CAD build for the part. Positions are in the model's coordinates, mm. A direction names the side the tool comes from. Round coordinates to 2 decimals unless told otherwise and drop trailing zeros. Loops run counter-clockwise (first coordinate to the right, second up) from the corner with the lowest first, then second, coordinate; pieces in that order, holes last. Notation, with made-up numbers: M -2,67 L 42,67 A30 cw 42,100 Z; hole C 12,83 d6. An arc over 180 degrees is marked long. Use one line per item in the form item = value.
from build123d import *

# Parameters (mm, degrees)
CROQUIS1_R              = 14
SALIENTE_EXTRUIR1_DEPTH = 3.5
CROQUIS2_R              = 17.2
SALIENTE_EXTRUIR2_DEPTH = 3.2
CROQUIS3_R              = 17.2
SALIENTE_EXTRUIR3_DEPTH = 3.2
CROQUIS4_R              = 1.5
CORTAR_EXTRUIR1_DEPTH   = 10.9
REDONDEO1_R             = 2
REDONDEO2_R             = 0.5


with BuildPart() as part:
    # Croquis1 → Saliente-Extruir1 (new body)
    with BuildSketch(Plane(origin=(0, 0, 0), x_dir=(1, 0, 0), z_dir=(0, 1, 0))):
        Circle(CROQUIS1_R)
    extrude(amount=SALIENTE_EXTRUIR1_DEPTH)

    # Croquis2 → Saliente-Extruir2 (add)
    with BuildSketch(Plane(origin=(0, 3.5, 0), x_dir=(1, 0, 0), z_dir=(0, 1, 0))):
        Circle(CROQUIS2_R)
    extrude(amount=SALIENTE_EXTRUIR2_DEPTH)

    # Croquis3 → Saliente-Extruir3 (add)
    with BuildSketch(Plane.XZ):
        Circle(CROQUIS3_R)
    extrude(amount=SALIENTE_EXTRUIR3_DEPTH)

    # Croquis4 → Cortar-Extruir1 (cut, through all)
    with BuildSketch(Plane.XZ.offset(3.2)):
        Circle(CROQUIS4_R)
    extrude(amount=-CORTAR_EXTRUIR1_DEPTH, mode=Mode.SUBTRACT)

    # Redondeo1
    redondeo1_edges = [part.edges().sort_by_distance(p)[0] for p in [
        (-17.2, 0, 0),
        (-17.2, 3.5, 0),
    ]]
    fillet(redondeo1_edges, radius=REDONDEO1_R)

    # Redondeo2
    redondeo2_edges = [part.edges().sort_by_distance(p)[0] for p in [
        (-14, 0, 0),
        (-14, 3.5, 0),
    ]]
    fillet(redondeo2_edges, radius=REDONDEO2_R)


solid = part.part
1. Probe line 1 along Y through (x, z) = (-7.5, -12.5); line 2 along Z through (x, y) = (0.5, 2.25); line 3 along Z through (x, y) = (0, -1). List the from-to ranges inside material, lowest first. Write a range as from..to.
Completed:
line_1 = -3.2..0, 3.5..6.7
line_2 = -13.99..-1.41, 1.41..13.99
line_3 = -16.93..-1.5, 1.5..16.93
2. Pull direction Z, two halves, no side cores. Call faces 1 (the face through (0, 0, -15)), 2 (the face through (-17.183, -2.592, 0.756)), 3 (the face through (-1.5, 1.68, 0.07)): +Z half, -Z half, draft (parallel to the pull), parting line (faces both ways), or undercut.
Completed:
face_1 = draft
face_2 = parting line
face_3 = undercut
3. Cut at B-B on z = 0. Write the cut outline in (x, y).
Completed:
outline = M -17.2,-3.2 L -1.5,-3.2 L -1.5,6.7 L -17.2,6.7 L -17.2,5.5 A2 ccw -15.2,3.5 L -14.5,3.5 A0.5 cw -14,3 L -14,0.5 A0.5 cw -14.5,0 L -15.2,0 A2 ccw -17.2,-2 Z; M 1.5,-3.2 L 17.2,-3.2 L 17.2,-2 A2 ccw 15.2,0 L 14.5,0 A0.5 cw 14,0.5 L 14,3 A0.5 cw 14.5,3.5 L 15.2,3.5 A2 ccw 17.2,5.5 L 17.2,6.7 L 1.5,6.7 Z
4. Cut at C-C on y = 6. Write the cut outline in (x, z).
Completed:
outline = C 0,0 d34.4; hole C 0,0 d3
5. Drop flat-ended pins along their axis: P1, Ø5, axis at y = -2, z = 10.5, coming from the +X side; P2, Ø5, axis at y = -1, z = 4.5, coming from the +X side; P3, Ø1, axis at y = 5.5, z = -12, coming from the -X side. Give the stop position or say it passes through.
Completed:
P1 = 15.23
P2 = 17.06
P3 = -12.79
6. Cut at A-A on x = 0. Write the cut outline in (y, z), and give its area (3 significant figures).
Completed:
outline = M -3.2,-17.2 L -2,-17.2 A2 ccw 0,-15.2 L 0,-14.5 A0.5 cw 0.5,-14 L 3,-14 A0.5 cw 3.5,-14.5 L 3.5,-15.2 A2 ccw 5.5,-17.2 L 6.7,-17.2 L 6.7,-1.5 L -3.2,-1.5 Z; M -3.2,1.5 L 6.7,1.5 L 6.7,17.2 L 5.5,17.2 A2 ccw 3.5,15.2 L 3.5,14.5 A0.5 cw 3,14 L 0.5,14 A0.5 cw 0,14.5 L 0,15.2 A2 ccw -2,17.2 L -3.2,17.2 Z
area = 285 mm2
7. Tool access for faces 4 (the face through (0, 3.5, 15)), 5 (the face through (0, 6.7, 4)): list every direction of +Z, -Z, +X, -X, +Y, -Y with a clear straight run to the whole face (end or side of a thin tool).
Completed:
face_4 = none
face_5 = +Z, -Z, +X, -X, +Y
